Source: CAD feature listing. Evaluate the final solid. Frame: model axes, mm. A direction names the side the tool comes from. Round coordinates to 2 decimals unless told otherwise and drop trailing zeros. Loops run counter-clockwise (first coordinate to the right, second up) from the corner with the lowest first, then second, coordinate; pieces in that order, holes last. Notation, with made-up numbers: M -20,58.25 L -2,58.25 A22 cw -2,91.25 Z; hole C 8.25,76 d1. An arc over 180 degrees is marked long. Write each question's results on one line, items separated by ' | '. Start each with the question number.
1. Section D-D on z = 16. Output: boundary loops of the cut face in (x, y), and give its area (3 significant figures).
2. Section B-B on z = 10.25. Output: boundary loops of the cut face in (x, y) (3 decimals).
3. Draft query along Z for faces 4 (the flat face through (0, 4, 15.24)), 5 (the flat face through (0, 3, 0)), 6 (the flat face through (0, 1, 6.096)), 7 (the flat face through (15.1, 4.5, 8.5)). Return one class per face: released by +Z, released by -Z, zero draft, split by the parting line, or undercut.
4. Contact query for a flat-ended pin moving along its axis: pin 1 Ø2 at (x, z) = (-6.5, 6.5) entering from +Y (3 decimals). Output: stop coordinate, or through.
5. Section C-C on x = -4. Output: boundary loops of the cut face in (y, z) (3 decimals), and give its area (3 significant figures).
6. Section A-A on y = 2.35. Output: boundary loops of the cut face in (x, z) (3 decimals), and give its area (3 significant figures).
7. Ray query, line 1 (Z direction, x = 0, y = 1.4); line 2 (Y direction, x = 6, z = 13.75) (3 decimals); line 3 (X direction, y = 2.95, z = 12.25). Return the intervals inside material, ascending.
8. Set-up query: faces 1 (the flat face through (0, 5.08, 16)), 2 (the cylindrical face through (8.507, 3.515, 8.491)), 3 (the cylindrical face through (4.444, 0.966, 8.58)). Return all of +Z, -Z, +X, -X, +Y, -Y with unobstructed straight access to the full face (end or side cutting, diameter ignored); none if empty.
from build123d import *

# Parameters (mm, degrees)
BOSS_EXTRUDE1_DEPTH   = 17.272
SKETCH2_OUTSIDE_W     = 40.918
SKETCH2_OUTSIDE_H     = 26.552
SKETCH2_OUTSIDE_W_2   = 31.63793758
SKETCH2_OUTSIDE_H_2   = 17.272
CUT_EXTRUDE1_DEPTH    = 3.175
CUT_EXTRUDE3_DEPTH    = 2.905
CHAMFER1_SIZE2        = 1.27
CHAMFER1_SIZE         = 0.990861631
CHAMFER1_EDGE_2_SIZE2 = 1.27
CHAMFER1_EDGE_2_SIZE  = 0.990861631


with BuildPart() as part:
    # Sketch1 → Boss-Extrude1 (new body)
    with BuildSketch(Plane.XY):
        Polygon((-13.97, 0), (13.97, 0), (15.81896879, 5.08), (-15.81896879, 5.08), align=None)
    extrude(amount=BOSS_EXTRUDE1_DEPTH)

    # Sketch2 outside → Cut-Extrude1 (cut)
    with BuildSketch(Plane(origin=(0, 5.08, 0), x_dir=(1, 0, 0), z_dir=(0, 1, 0))):
        with Locations((0, -8.636)):
            Rectangle(SKETCH2_OUTSIDE_W, SKETCH2_OUTSIDE_H)
        with Locations((0, -8.636)):
            Rectangle(SKETCH2_OUTSIDE_W_2, SKETCH2_OUTSIDE_H_2, mode=Mode.SUBTRACT)
        with BuildLine():
            Line((1.905, -15.24), (-1.905, -15.24))
            ThreePointArc((-1.905, -15.24), (-8.509, -8.636), (-1.905, -2.032))
            Line((-1.905, -2.032), (1.905, -2.032))
            ThreePointArc((1.905, -2.032), (8.509, -8.636), (1.905, -15.24))
        make_face()
    extrude(amount=-CUT_EXTRUDE1_DEPTH, mode=Mode.SUBTRACT)

    # Sketch4 → Cut-Extrude3 (cut, through all)
    with BuildSketch(Plane(origin=(0, 1.905, 0), x_dir=(1, 0, 0), z_dir=(0, 1, 0))):
        with BuildLine():
            Line((1.905, -11.176), (-1.905, -11.176))
            ThreePointArc((-1.905, -11.176), (-4.445, -8.636), (-1.905, -6.096))
            Line((-1.905, -6.096), (1.905, -6.096))
            ThreePointArc((1.905, -6.096), (4.445, -8.636), (1.905, -11.176))
        make_face()
    extrude(amount=-CUT_EXTRUDE3_DEPTH, mode=Mode.SUBTRACT)

    # Chamfer1
    chamfer1_edges = [part.edges().sort_by_distance(p)[0] for p in [
        (-15.81896879, 5.08, 8.636),
    ]]
    chamfer(chamfer1_edges, length=CHAMFER1_SIZE, length2=CHAMFER1_SIZE2)

    # Chamfer1 edge 2
    chamfer1_edge_2_edges = [part.edges().sort_by_distance(p)[0] for p in [
        (15.81896879, 5.08, 8.636),
    ]]
    chamfer(chamfer1_edge_2_edges, length=CHAMFER1_EDGE_2_SIZE, length2=CHAMFER1_EDGE_2_SIZE2)


solid = part.part
Taken from the geometry:
1) outline: M -15.48,4.15 L -13.97,0 L 13.97,0 L 15.38,3.89 L 14.83,5.08 L -14.55,5.08 Z | area: 150 mm^2
2) outline: M -15.48,4.149 L -13.97,0 L -3.866,0 L -3.866,1.905 L -8.309,1.905 L -8.309,5.08 L -14.549,5.08 Z; M 3.866,0 L 13.97,0 L 15.385,3.887 L 14.828,5.08 L 8.309,5.08 L 8.309,1.905 L 3.866,1.905 Z
3) face 4: undercut | face 5: released by -Z | face 6: undercut | face 7: zero draft
4) pin 1: y = 1.905
5) outline: M 0,0 L 5.08,0 L 5.08,2.373 L 1.905,2.373 L 1.905,7.2 L 0,7.2 Z; M 0,10.072 L 1.905,10.072 L 1.905,14.899 L 5.08,14.899 L 5.08,17.272 L 0,17.272 Z | area: 42.5 mm^2
6) outline: M -14.825,0 L 14.825,0 L 14.825,17.272 L -14.825,17.272 Z; hole M -1.905,2.032 L 1.905,2.032 A6.604 ccw 1.905,15.24 L -1.905,15.24 A6.604 ccw Z | area: 325 mm^2
7) line 1: 0 to 6.1, 11.18 to 17.27 | line 2: 0 to 1.905 | line 3: -15.04 to -7.43, 7.43 to 15.04
8) face 1: +Z, -Z, +X, -X, +Y | face 2: +Y | face 3: +Y, -Y
